Verification items for this drawing (mm, ordinates from the low corner). A direction names the side the tool comes from. Coordinates: 2 decimals unless noted, no trailing zeros. Write each loop counter-clockwise with the first axis right and the second up, starting at its lowest first coordinate (ties: lowest second). Pieces come first, ordered by that corner, then holes. Notation, with made-up numbers: (86.5, -22.5) -> (103.5, -22.5) arc R28 cw to (103.5, 0.5) -> close; hole circle Ø8 at (80.5, -27). An arc over 180 degrees is marked (long way). Answer as CSV lines item,"result".
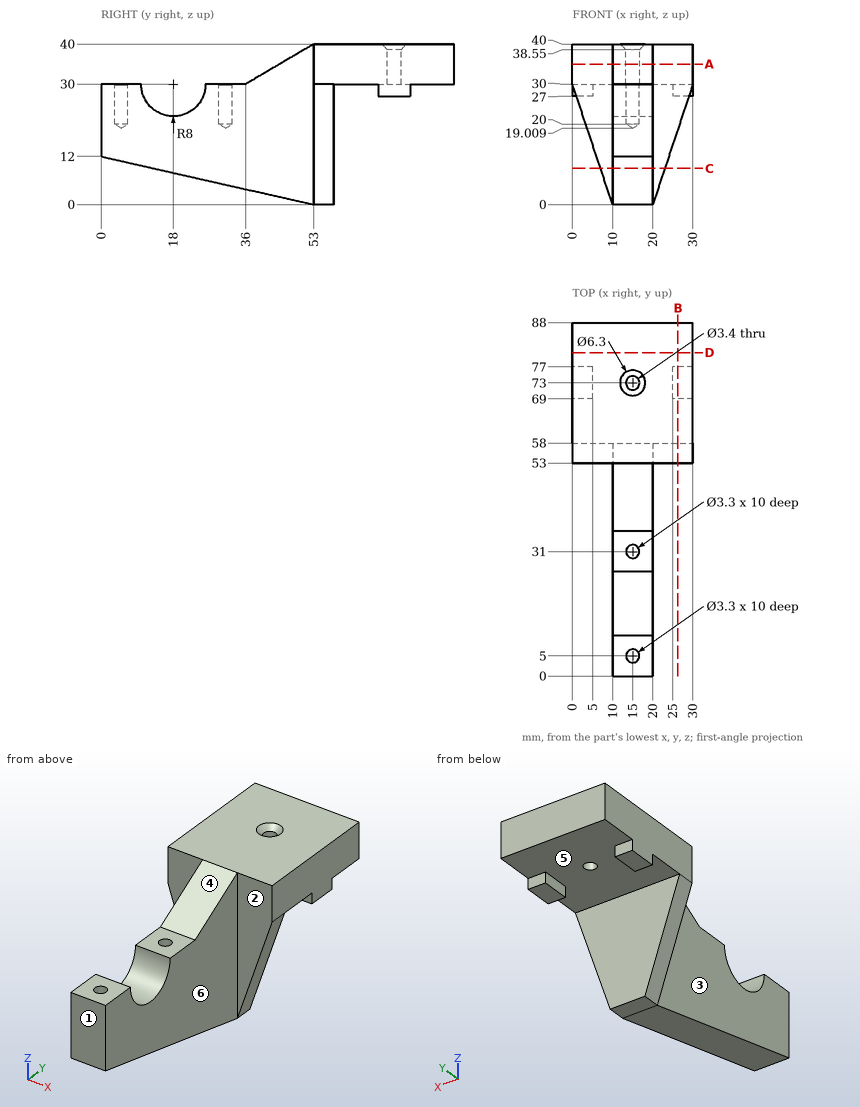
Item 1: Depth check by flat-ended pin: pin 1 Ø3 at (x, y) = (15, 31) entering from +Z; pin 2 Ø1 at (y, z) = (43.5, 28) entering from +X; pin 3 Ø8 at (x, z) = (11.5, 25) entering from +Y; pin 4 Ø12 at (x, z) = (7, 17) entering from -Y. Enter the tip coordinate at first touch or a pass-through.
Responses:
pin 1,"stops at z = 19.91"
pin 2,"stops at x = 20"
pin 3,"stops at y = 58"
pin 4,"stops at y = 0"
Item 2: Set-up check for the marked faces 1, 2 and 3: record each of +Z, -Z, +X, -X, +Y, -Y from which the full face is reachable in a straight line by a thin tool's end or side.
Responses:
face 1,"+Z, -Z, +X, -X, -Y"
face 2,"+Z, -Z, +X, -Y"
face 3,"+Z, -Z, -X, -Y"
Item 3: Cross-section at C-C, the plane z = 9. Record the cut outline in (x, y).
Responses:
outline,"(7, 53) -> (10, 53) -> (10, 13.25) -> (20, 13.25) -> (20, 53) -> (23, 53) -> (23, 58) -> (7, 58) -> close"
Item 4: Cross-section at A-A, the plane z = 35. Record the cut outline in (x, y).
Responses:
outline,"(0, 53) -> (10, 53) -> (10, 44.5) -> (20, 44.5) -> (20, 53) -> (30, 53) -> (30, 88) -> (0, 88) -> close; hole circle Ø3.4 at (15, 73)"
Item 5: Thickness scan on probe 1 along X at (y, z) = (73, 32); probe 2 along Y at (x, z) = (6.5, 23.5); probe 3 along X at (y, z) = (33.5, 26). Record the ranges inside material, lowest first.
Responses:
probe 1,"x = 0 to 13.3, 16.7 to 30"
probe 2,"y = 53 to 58"
probe 3,"x = 10 to 20"
Item 6: Cross-section at D-D, the plane y = 80.5. Record the cut outline in (x, z).
Responses:
outline,"(0, 30) -> (30, 30) -> (30, 40) -> (0, 40) -> close"
Item 7: Release check for a two-part mould opening along X. For the marked faces 4, 5 and 6 record: +X half, -X half, draft (parallel to the pull), parting line (faces both ways), or undercut.
Responses:
face 4,"draft"
face 5,"undercut"
face 6,"+X half"
Item 8: Cross-section at B-B, the plane x = 26.25. Record the cut outline in (y, z), plus the area to 3 significant figures.
Responses:
outline,"(53, 18.75) -> (58, 18.75) -> (58, 30) -> (69, 30) -> (69, 27) -> (77, 27) -> (77, 30) -> (88, 30) -> (88, 40) -> (53, 40) -> close"
area,"430 mm2"
